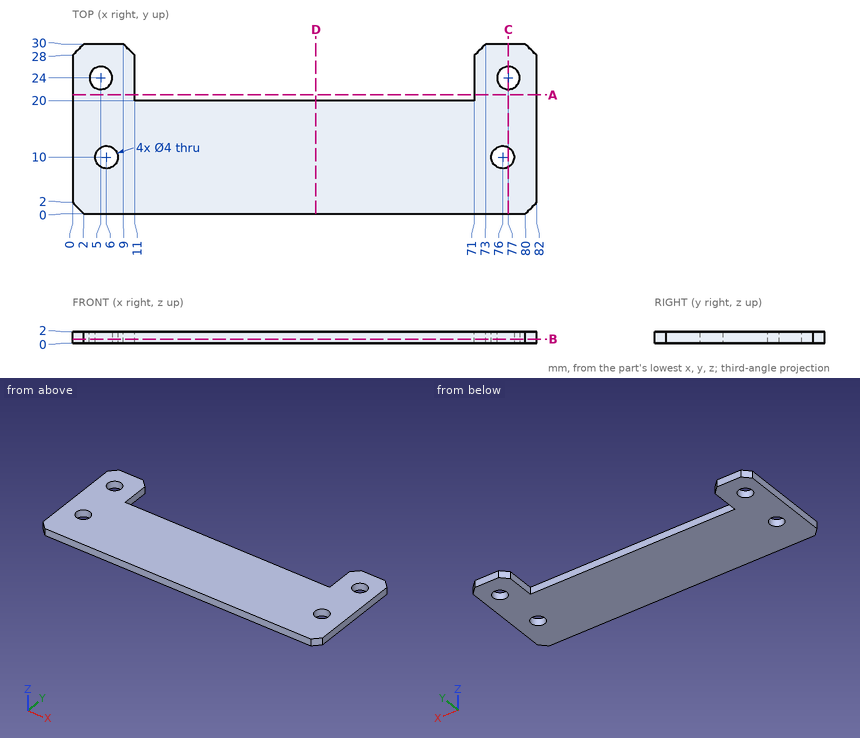
Input: dimensioned drawing with shaded views. Units: mm. Origin: part minimum x, y, z. Coordinates: 2 decimals unless noted, no trailing zeros. Loops run counter-clockwise (first coordinate to the right, second up) from the corner with the lowest first, then second, coordinate; pieces in that order, holes last. Notation, with made-up numbers: M 66,50.25 L 87,50.25 A13 cw 87,65.25 Z; hole C 32,-18.5 d10. An arc over 180 degrees is marked long. Use a Markdown table: item, result. Add a question column.
Q1. Section query C-C, the plane x = 77. Return loops of the section in (y, z).
Q2. Section query B-B, the plane z = 0.7. Return loops of the section in (x, y).
Q3. Section query D-D, the plane x = 43. Return loops of the section in (y, z).
Q4. Section query A-A, the plane y = 21. Return loops of the section in (x, z), and give its area (3 significant figures).
Q5. First-contact query: pin 1 (0.6 mm diameter, centred on x = 35, z = 1, fed in from +Y); pin 2 (3.5 mm diameter, centred on x = 5, y = 24, fed in from +Z). Flat tips, straight axial feed; report the tip coordinate or a pass-through.
Q6. Material intervals for L1, parallel to Y at x = 77, z = 1.3; L2, parallel to Y at x = 76, z = 0.6; L3, parallel to X at y = 10.5, z = 0.25, sorted ascending.
Result:
| question | item | result |
|---|---|---|
| 1 | outline | M 0,0 L 8.27,0 L 8.27,2 L 0,2 Z; M 11.73,0 L 22,0 L 22,2 L 11.73,2 Z; M 26,0 L 30,0 L 30,2 L 26,2 Z |
| 2 | outline | M 0,2 L 2,0 L 80,0 L 82,2 L 82,28 L 80,30 L 73,30 L 71,28 L 71,20 L 11,20 L 11,28 L 9,30 L 2,30 L 0,28 Z; hole C 5,24 d4; hole C 6,10 d4; hole C 76,10 d4; hole C 77,24 d4 |
| 3 | outline | M 0,0 L 20,0 L 20,2 L 0,2 Z |
| 4 | outline | M 0,0 L 11,0 L 11,2 L 0,2 Z; M 71,0 L 82,0 L 82,2 L 71,2 Z |
| 4 | area | 44.0 mm2 |
| 5 | pin 1 | stops at y = 20 |
| 5 | pin 2 | passes through |
| 6 | L1 | y = 0 to 8.27, 11.73 to 22, 26 to 30 |
| 6 | L2 | y = 0 to 8, 12 to 22.27, 25.73 to 30 |
| 6 | L3 | x = 0 to 4.06, 7.94 to 74.06, 77.94 to 82 |
